Autodesk Inventor part; units mm, degrees
ref_plane "YZ Plane" through (0, 0, 0) normal (1, 0, 0) x (0, 1, 0)
ref_plane "XZ Plane" through (0, 0, 0) normal (0, 1, 0) x (-1, 0, 0)
ref_plane "XY Plane" through (0, 0, 0) normal (0, 0, 1) x (1, 0, 0)
sketch "スケッチ1" plane through (0, 0, 0) normal (0, 0, 1) x (1, 0, 0)
  circle A0 centre (0, 0) radius 2.5
  dimension "d0" = 5
extrude "押し出し1" add sketch "スケッチ1" along normal blind 34
sketch "スケッチ2" plane through (0, 0, 34) normal (0, 0, 1) x (1, 0, 0)
  circle A0 centre (0, 0) radius 1.5
  dimension "d3" = 3
extrude "押し出し2" cut sketch "スケッチ2" against normal blind 6
sketch "スケッチ3" plane through (0, 0, 0) normal (0, 1, 0) x (-1, 0, 0)
  line L0 (2.5, 0) -> (2.5, 34)
  line L1 (2.5, 23.9) -> (2.5, 26.9)
  line L2 (2.5, 26.9) -> (1.5, 26.9)
  line L3 (1.5, 26.9) -> (1.5, 20.9)
  line L4 (1.5, 20.9) -> (2.5, 20.9)
  line L5 (2.5, 20.9) -> (2.5, 23.9)
  point P0 (0, 0)
  dimension "d8" = 3
  dimension "d9" = 1
  dimension "d10" = 6
extrude "押し出し3" cut sketch "スケッチ3" along normal mid plane 10
thread "ねじ2"
properties part number "shaft_34mm_Φ5" material "アルミニウム 7075"
Design review of the part built by this model. Coordinates are the model's own, in mm. A direction names the side the tool comes from. Round coordinates to 2 decimals unless told otherwise and drop trailing zeros. Write each loop counter-clockwise with the first axis right and the second up, starting at its lowest first coordinate (ties: lowest second). Pieces come first, ordered by that corner, then holes. Notation, with made-up numbers: (-14, 84) -> (14, 84) arc R19 cw to (14, 98) -> close; hole circle Ø8 at (67.5, 51). An arc over 180 degrees is marked (long way). Answer in a Markdown table with one row per item.
Q1. Take a section at C-C, the plane x = -0.3. State the section outline as (y, z) points, then the cut area to 3 significant figures.
The answers:
| item | result |
|---|---|
| outline | (-2.48, 0) -> (2.48, 0) -> (2.48, 34) -> (1.47, 34) -> (1.47, 28) -> (-1.47, 28) -> (-1.47, 34) -> (-2.48, 34) -> close |
| area | 151 mm² |
Q2. For faces 1 (the face through (0, 0, 0)), 2 (the face through (-2, 0, 26.9)), 3 (the face through (0, 0, 28)), list the 3-axis set-ups (+Z, -Z, +X, -X, +Y, -Y) from which the entire face can be reached by the end or side of a thin tool; tool diameter is ignored.
The answers:
| item | result |
|---|---|
| face 1 | -Z, +X, -X, +Y, -Y |
| face 2 | -X, +Y, -Y |
| face 3 | +Z |
Q3. To check wall thickness, follow L1, parallel to Z at x = -2, y = 0.6; L2, parallel to Y at x = 0, z = 29.2; L3, parallel to X at y = 0.1, z = 26. State the ranges of each line that lie inside material, in increasing order. Write a range as [from, to].
The answers:
| item | result |
|---|---|
| L1 | [0, 20.9], [26.9, 34] |
| L2 | [-2.5, -1.5], [1.5, 2.5] |
| L3 | [-1.5, 2.5] |
Q4. Clearance check with flat-ended pins moving along their axes: pin 1 Ø2.5 at (x, y) = (0, 0) entering from +Z; pin 2 Ø2 at (x, z) = (2, 22.5) entering from -Y; pin 3 Ø1.5 at (x, z) = (-1.5, 13.5) entering from -Y. State where each tip first meets the part, or that it passes through.
The answers:
| item | result |
|---|---|
| pin 1 | z = 28 |
| pin 2 | y = -2.29 |
| pin 3 | y = -2.38 |
Q5. Take a section at A-A, the plane z = 31. State the section outline as (x, y) points.
The answers:
| item | result |
|---|---|
| outline | circle Ø5 at (0, 0); hole circle Ø3 at (0, 0) |
Q6. Take a section at B-B, the plane y = 0. State the section outline as (x, z) points, then the cut area to 3 significant figures.
The answers:
| item | result |
|---|---|
| outline | (-2.5, 0) -> (2.5, 0) -> (2.5, 34) -> (1.5, 34) -> (1.5, 28) -> (-1.5, 28) -> (-1.5, 34) -> (-2.5, 34) -> (-2.5, 26.9) -> (-1.5, 26.9) -> (-1.5, 20.9) -> (-2.5, 20.9) -> close |
| area | 146 mm² |
Q7. Take a section at D-D, the plane z = 8. State the section outline as (x, y) points, then the cut area to 3 significant figures.
The answers:
| item | result |
|---|---|
| outline | circle Ø5 at (0, 0) |
| area | 19.6 mm² |
Q8. Draft analysis for pull direction Z (two halves, no side actions). For faces 4 (the face through (2, 0, 34)), 5 (the face through (-2, 0, 20.9)), 6 (the face through (-1.5, 0.07, 31.04)), state which applies: +Z half, -Z half, draft (parallel to the pull), parting line (faces both ways), or undercut.
The answers:
| item | result |
|---|---|
| face 4 | +Z half |
| face 5 | undercut |
| face 6 | draft |
